```python
from build123d import *

# Parameters (mm, degrees)
BOSS_EXTRUDE1_DEPTH              = 4.7625
SKETCH3_R                        = 9.525
CUT_EXTRUDE1_DEPTH               = 5.7625
F_6_CLEARANCE_HOLE1_D            = 4.3053
F_23_64_0_35938_DIAMETER_HOLE1_D = 9.128252
FILLET1_R                        = 1.5875


with BuildPart() as part:
    # Sketch1 → Boss-Extrude1 (new body)
    with BuildSketch(Plane.XY):
        with BuildLine():
            Line((-40.9575, 29.810203833), (-40.9575, 27.270203833))
            ThreePointArc((-40.9575, 27.270203833), (-42.352403955, 23.902607788), (-45.72, 22.507703833))
            Line((-45.72, 22.507703833), (-48.26, 22.507703833))
            Line((-48.26, 22.507703833), (-48.26, 1.870203833))
            Line((-48.26, 1.870203833), (-85.725, 1.870203833))
            Line((-85.725, 1.870203833), (-85.725, -38.769796167))
            Line((-85.725, -38.769796167), (85.725, -38.769796167))
            Line((85.725, -38.769796167), (85.725, 1.870203833))
            Line((85.725, 1.870203833), (48.26, 1.870203833))
            Line((48.26, 1.870203833), (48.26, 29.810203833))
            Line((48.26, 29.810203833), (21.2725, 29.810203833))
            Line((21.2725, 29.810203833), (21.2725, 27.270203833))
            ThreePointArc((21.2725, 27.270203833), (16.51, 22.507703833), (11.7475, 27.270203833))
            Line((11.7475, 27.270203833), (11.7475, 29.810203833))
            Line((11.7475, 29.810203833), (-40.9575, 29.810203833))
        make_face()
    extrude(amount=BOSS_EXTRUDE1_DEPTH)

    # Sketch3 → Cut-Extrude1 (cut, through all)
    with BuildSketch(Plane.XY.offset(4.7625)):
        with Locations((73.025, -15.909796167)):
            Circle(SKETCH3_R)
        with Locations((42.8625, -15.909796167)):
            Circle(SKETCH3_R)
        with Locations((12.7, -15.909796167)):
            Circle(SKETCH3_R)
        with Locations((-15.875, -15.909796167)):
            Circle(SKETCH3_R)
        with Locations((-44.45, -15.909796167)):
            Circle(SKETCH3_R)
        with Locations((-74.6125, -15.909796167)):
            Circle(SKETCH3_R)
        with Locations((34.29, 13.617703833)):
            Circle(SKETCH3_R)
        with Locations((6.35, 13.617703833)):
            Circle(SKETCH3_R)
        with Locations((-24.13, 13.617703833)):
            Circle(SKETCH3_R)
    extrude(amount=-CUT_EXTRUDE1_DEPTH, mode=Mode.SUBTRACT)

    # #6 Clearance Hole1 (through all)
    with Locations(Plane.XY.offset(4.7625)):
        with Locations((57.15, -8.924796167), (21.59, 19.015203833), (-60.96, -8.924796167)):
            Hole(F_6_CLEARANCE_HOLE1_D / 2)

    # 23/64 (0.35938) Diameter Hole1 (through all)
    with Locations(Plane.XY.offset(4.7625)):
        with Locations((57.15, -31.149796167), (-60.96, -31.149796167)):
            Hole(F_23_64_0_35938_DIAMETER_HOLE1_D / 2)

    # Fillet1
    fillet1_edges = [part.edges().sort_by_distance(p)[0] for p in [
        (11.7475, 29.810203833, 2.38125),
        (21.2725, 29.810203833, 2.38125),
        (48.26, 29.810203833, 2.38125),
        (48.26, 1.870203833, 2.38125),
        (85.725, 1.870203833, 2.38125),
        (85.725, -38.769796167, 2.38125),
        (-85.725, -38.769796167, 2.38125),
        (-85.725, 1.870203833, 2.38125),
        (-48.26, 1.870203833, 2.38125),
        (-48.26, 22.507703833, 2.38125),
        (-40.9575, 29.810203833, 2.38125),
    ]]
    fillet(fillet1_edges, radius=FILLET1_R)


solid = part.part
```
Verification items for the finished model (mm, model axes). A direction names the side the tool comes from. Give positions to 0.01 mm unless a question says otherwise; leave off trailing zeros. Write each loop counter-clockwise with the first axis right and the second up, starting at its lowest first coordinate (ties: lowest second). Pieces come first, ordered by that corner, then holes. Notation, with made-up numbers: M 39.25,10.5 L 45.25,10.5 A8 ccw 45.25,16.5 Z; hole C 68.25,-17 d6. An arc over 180 degrees is marked long. One line per question, with ' | ' between items.
1) Section check A-A on x = 57.15. Enter the section's corners in (y, z).
Result:
outline: M -38.77,0 L -35.71,0 L -35.71,4.76 L -38.77,4.76 Z; M -26.59,0 L -11.08,0 L -11.08,4.76 L -26.59,4.76 Z; M -6.77,0 L 1.87,0 L 1.87,4.76 L -6.77,4.76 Z
2) Mould release check, pull along X, two halves, no side actions. Record for faces 1 (the flat face through (85.725, -19, 2)), 2 (the flat face through (-14, 29.81, 2)), 3 (the cylindrical face through (-33.646, 14.037, 2.415)): released by +X, released by -X, zero draft, split by the parting line, or undercut.
Result:
face 1: released by +X | face 2: zero draft | face 3: undercut
3) Section check C-C on y = -19.5. Enter the section's corners in (x, z) (1 decimal), plus the area to 3 significant figures.
Result:
outline: M -85.7,0 L -83.4,0 L -83.4,4.8 L -85.7,4.8 Z; M -65.8,0 L -53.3,0 L -53.3,4.8 L -65.8,4.8 Z; M -35.6,0 L -24.7,0 L -24.7,4.8 L -35.6,4.8 Z; M -7.1,0 L 3.9,0 L 3.9,4.8 L -7.1,4.8 Z; M 21.5,0 L 34,0 L 34,4.8 L 21.5,4.8 Z; M 51.7,0 L 64.2,0 L 64.2,4.8 L 51.7,4.8 Z; M 81.8,0 L 85.7,0 L 85.7,4.8 L 81.8,4.8 Z | area: 312 mm2
4) Thickness scan on line 1 along X through (y, z) = (8.5, 3.9); line 2 along Y through (x, z) = (-24.5, 2.15); line 3 along Y through (x, z) = (57, 2.25). Record the ranges inside material, lowest first. Write a range as [from, to].
Result:
line 1: x = [-48.26, -32.16], [-16.1, -1.68], [14.38, 26.26], [42.32, 48.26] | line 2: y = [-38.77, -19.95], [-11.87, 4.1], [23.14, 29.81] | line 3: y = [-38.77, -35.71], [-26.59, -11.07], [-6.78, 1.87]
5) Set-up check for faces 4 (the flat face through (-85.725, -18, 2)), 5 (the flat face through (67, 1.87, 2)), 6 (the flat face through (-67, 1.87, 2)): record each of +Z, -Z, +X, -X, +Y, -Y from which the full face is reachable in a straight line by a thin tool's end or side.
Result:
face 4: +Z, -Z, -X, +Y, -Y | face 5: +Z, -Z, +X, +Y | face 6: +Z, -Z, -X, +Y
6) Section check D-D on x = 6.35. Enter the section's corners in (y, z).
Result:
outline: M -38.77,0 L -23.01,0 L -23.01,4.76 L -38.77,4.76 Z; M -8.81,0 L 4.09,0 L 4.09,4.76 L -8.81,4.76 Z; M 23.14,0 L 29.81,0 L 29.81,4.76 L 23.14,4.76 Z
7) Section check B-B on y = 7.5. Enter the section's corners in (x, z), plus the area to 3 significant figures.
Result:
outline: M -48.26,0 L -31.43,0 L -31.43,4.76 L -48.26,4.76 Z; M -16.83,0 L -0.95,0 L -0.95,4.76 L -16.83,4.76 Z; M 13.65,0 L 26.99,0 L 26.99,4.76 L 13.65,4.76 Z; M 41.59,0 L 48.26,0 L 48.26,4.76 L 41.59,4.76 Z | area: 251 mm2
8) Gauge pin test, flat ends, axial feed: pin 1 Ø2.5 at (x, z) = (73.5, 3) entering from +Y; pin 2 Ø15 at (x, y) = (-24.13, 13.62) entering from -Z. Record the tip position at first contact, or that the pin passes through.
Result:
pin 1: stops at y = 1.87 | pin 2: passes through
